from build123d import *

# Parameters (mm, degrees)
F0_W     = 3
F0_H     = 3
F1_DEPTH = 3
F3_DEPTH = 4.5
F4_SIZE2 = 0.803838
F4_SIZE  = 2.99999


# Not quite as in the source:
# - a fillet or chamfer is up to 0.001 mm smaller than in the source, because OpenCascade refuses the exact size


with BuildPart() as f1:
    # F0 (on Top) → F1 (new body)
    with BuildSketch(Plane.XY):
        with BuildLine():
            Line((-6.5, 25.75), (-10.95, 25.75))
            Line((-10.95, 25.75), (-10.95, 22.75))
            Line((-10.95, 22.75), (-10.95, -23.75))
            ThreePointArc((-10.95, -23.75), (-10.3642135624, -25.1642135624), (-8.95, -25.75))
            Line((-8.95, -25.75), (8.95, -25.75))
            ThreePointArc((8.95, -25.75), (10.3642135624, -25.1642135624), (10.95, -23.75))
            Line((10.95, -23.75), (10.95, 22.75))
            Line((10.95, 22.75), (10.95, 25.75))
            Line((10.95, 25.75), (6.5, 25.75))
            Line((6.5, 25.75), (6.5, 6.75))
            ThreePointArc((6.5, 6.75), (6.2071067812, 6.0428932188), (5.5, 5.75))
            ThreePointArc((5.5, 5.75), (4.7928932188, 6.0428932188), (4.5, 6.75))
            Line((4.5, 6.75), (4.5, 25.75))
            Line((4.5, 25.75), (-4.5, 25.75))
            Line((-4.5, 25.75), (-4.5, 6.75))
            ThreePointArc((-4.5, 6.75), (-4.7928932188, 6.0428932188), (-5.5, 5.75))
            ThreePointArc((-5.5, 5.75), (-6.2071067812, 6.0428932188), (-6.5, 6.75))
            Line((-6.5, 6.75), (-6.5, 25.75))
        make_face()
        with Locations((-12.45, 24.25)):
            Rectangle(F0_W, F0_H)
        with Locations((12.45, 24.25)):
            Rectangle(F0_W, F0_H)
    extrude(amount=F1_DEPTH)

    # F2 (on Right) → F3 (join, symmetric)
    with BuildSketch(Plane.YZ):
        Polygon((-25.75, 0), (25.75, 0), (30.25, 4.5), align=None)
    extrude(amount=F3_DEPTH, both=True)

    # F4 (size 3 and 0.8038475773 in the source; OpenCascade refuses exactly that, so slightly less here)
    f4_edges = [f1.edges().sort_by_distance(p)[0] for p in [
        (0, -25.75, 0),
    ]]
    f4_side = f1.faces().sort_by_distance((0, -25.75, 1.5))[0]
    chamfer(f4_edges, length=F4_SIZE, length2=F4_SIZE2, reference=f4_side)


solid = f1.part
Read the model definition and answer for the solid it produces. Units are mm, in the model's axes. A direction names the side the tool comes from. Round coordinates to 2 decimals unless told otherwise and drop trailing zeros. Loops run counter-clockwise (first coordinate to the right, second up) from the corner with the lowest first, then second, coordinate; pieces in that order, holes last.
Q1. Section A-A on y = 9 is taken. Give the number of separate pieces and of enclosed holes in the cut face, and give its area (3 significant figures).
Q2. Consider probe 1 along X at (y, z) = (17.5, 2.45); probe 2 along X at (y, z) = (9.5, 1.95); probe 3 along Z at (x, y) = (-8.75, -16.5). Determine where each line is inside the solid, lowest interval first.
Q3. Each of these flat-tipped pins is pushed along its axis until it touches: pin 1 (1.5 mm diameter, centred on x = 8.5, z = 2, fed in from +Y); pin 2 (4 mm diameter, centred on x = 4, y = 23.5, fed in from -Z); pin 3 (8 mm diameter, centred on x = 6.5, y = -3, fed in from +Z); pin 4 (2 mm diameter, centred on y = 17.5, z = 1, fed in from +X). Where does it stop, or does it pass through?
Q4. Which of the six approach directions +Z, -Z, +X, -X, +Y, -Y give full straight-line access (tool end or side, diameter ignored) to faces 1 (the face through (4.5, 18, 2)), 2 (the face through (-10.542, -0.826, 1.479)), 3 (the face through (10.542, -0.175, 1.479))?
Q5. Section D-D on z = 1.55 is taken. Write down the section's boundary in (x, y), and give its area (3 significant figures).
Output:
1. separate pieces: 3
1. enclosed holes: 0
1. area: 51.3 mm2
2. probe 1: x = -10.8 to -6.5, -4.5 to 4.5, 6.5 to 10.8
2. probe 2: x = -10.67 to -6.5, -4.5 to 4.5, 6.5 to 10.67
2. probe 3: z = 0 to 3
3. pin 1: stops at y = 25.75
3. pin 2: stops at z = 0
3. pin 3: stops at z = 3
3. pin 4: stops at x = 10.68
4. face 1: +Z, -Z, +Y
4. face 2: -Z, -X, -Y
4. face 3: -Z, +X, -Y
5. outline: (-13.95, 22.75) - (-10.56, 22.75) - (-10.56, -23.75) arc R1.61 ccw to (-8.95, -25.36) - (8.95, -25.36) arc R1.61 ccw to (10.56, -23.75) - (10.56, 22.75) - (13.95, 22.75) - (13.95, 25.75) - (6.5, 25.75) - (6.5, 6.75) arc R1 cw to (4.5, 6.75) - (4.5, 27.3) - (-4.5, 27.3) - (-4.5, 6.75) arc R1 cw to (-6.5, 6.75) - (-6.5, 25.75) - (-13.95, 25.75) - close
5. area: 1,030 mm2
